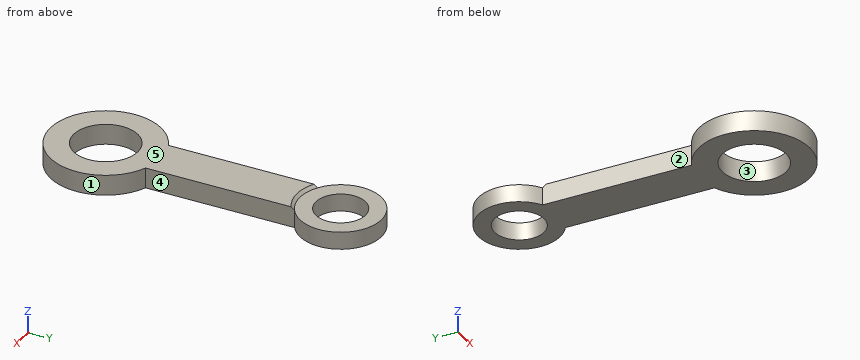
Autodesk Inventor part; units mm, degrees
ref_plane "YZ Plane" through (0, 0, 0) normal (1, 0, 0) x (0, 1, 0)
ref_plane "XZ Plane" through (0, 0, 0) normal (0, 1, 0) x (-1, 0, 0)
ref_plane "XY Plane" through (0, 0, 0) normal (0, 0, 1) x (1, 0, 0)
sketch "Sketch1" plane through (0, 0, 0) normal (0, 0, 1) x (1, 0, 0)
  line L0 (0, 0) -> (0, 80) construction
  circle A0 centre (0, 0) radius 11
  circle A1 centre (0, 80) radius 8.5
  line L1 (7.5, 17.4571) -> (-7.5, 17.4571)
  line L2 (-7.5, 17.4571) -> (-7.5, 68.1784)
  line L3 (-7.5, 68.1784) -> (7.5, 68.1784)
  line L4 (7.5, 68.1784) -> (7.5, 17.4571)
  line L5 (7.5, 17.4571) -> (-7.5, 68.1784) construction
  line L6 (-7.5, 17.4571) -> (7.5, 68.1784) construction
  arc A2 (7.5, 68.1784) -> (-7.5, 68.1784) centre (0, 80) ccw
  arc A3 (-7.5, 17.4571) -> (7.5, 17.4571) centre (0, 0) ccw
  point P0 (0, 42.8177)
  point P1 (0, 42.8177)
  dimension "d0" = 22
  dimension "d1" = 17
  dimension "d2" = 80
  dimension "d3" = 5.5
  dimension "d4" = 8
  dimension "d5" = 15
extrude "Extrusion1" add sketch "Sketch1" along normal blind 7
sketch "Sketch2" plane through (0, 0, 7) normal (0, 0, 1) x (1, 0, 0)
  circle A0 centre (0, 80) radius 8.5
  arc A1 (7.5, 68.1784) -> (-7.5, 68.1784) centre (0, 80) ccw
  circle A2 centre (0, 80) radius 14
extrude "Extrusion2" cut sketch "Sketch2" against normal blind 1
chamfer "Chamfer1" distance 1 angle 45 1 edges at (0, 66, 7)
properties part number "con rod"
Build history of the part. All positions in model axes, mm. Face numbers are marked on the shaded views. A direction names the side the tool comes from. Give positions to 0.01 mm unless a question says otherwise; leave off trailing zeros. Order: outer loops, then holes, each group sorted by start corner. A loop starts at its lowest first (then second) coordinate and runs counter-clockwise, first axis right, second up. Notation, with made-up numbers: M -20,75.5 L 2,75.5 A18 cw 2,99.5 Z; hole C 21,15.5 d8. An arc over 180 degrees is marked long. Put each result on its own line as item: value.
Item 1: Slice it at B-B, the plane y = 80. Write the cut outline in (x, z).
From the geometry:
outline: M -14,0 L -8.5,0 L -8.5,6 L -14,6 Z; M 8.5,0 L 14,0 L 14,6 L 8.5,6 Z
Item 2: Slice it at A-A, the plane x = 0. Give the number of separate pieces and of enclosed holes in the cut face, plus the area to 4 significant figures.
From the geometry:
separate pieces: 3
enclosed holes: 0
area: 506.5 mm2
Item 3: Slice it at C-C, the plane z = 3.5. Write the cut outline in (x, y).
From the geometry:
outline: M -7.5,17.46 A19 ccw long 7.5,17.46 L 7.5,68.18 A14 ccw long -7.5,68.18 Z; hole C 0,0 d22; hole C 0,80 d17
Item 4: 3-axis set-ups, long thin cutter, end or side, ignore diameter. For the marked faces 1 and 2: which of +Z, -Z, +X, -X, +Y, -Y reach the whole face in a straight line?
From the geometry:
face 1: +Z, -Z
face 2: +Z, -Z, -X
Item 5: Probe line 1 (Y direction, x = 0, z = 1.85); line 2 (Y direction, x = 7, z = 5); line 3 (X direction, y = 32, z = 1.75). List the from-to ranges inside material, lowest first. Write a range as [from, to].
From the geometry:
line 1: y = [-19, -11], [11, 71.5], [88.5, 94]
line 2: y = [-17.66, -8.49], [8.49, 75.18], [84.82, 92.12]
line 3: x = [-7.5, 7.5]
Item 6: Flat gauge pins, fed straight in: pin 1 Ø1.5 at (x, z) = (-1, 4.5) entering from +Y; pin 2 Ø10 at (x, y) = (-8, 35) entering from -Z; pin 3 Ø2 at (y, z) = (34.5, 5) entering from +X; pin 4 Ø3 at (x, z) = (13.5, 2) entering from -Y. Where does each tip first touch, or does it go through?
From the geometry:
pin 1: stops at y = 94
pin 2: stops at z = 0
pin 3: stops at x = 7.5
pin 4: stops at y = -14.73
Item 7: Slice it at D-D, the plane x = -12.5. Write the cut outline in (y, z), plus the area to 3 significant figures.
From the geometry:
outline: M -14.31,0 L 14.31,0 L 14.31,7 L -14.31,7 Z; M 73.7,0 L 86.3,0 L 86.3,6 L 73.7,6 Z
area: 276 mm2
Item 8: Two-plate mould, pull along Y, no slides. Class the marked faces 3, 4 and 5: +Y half, -Y half, draft (parallel to the pull), parting line (faces both ways), or undercut.
From the geometry:
face 3: undercut
face 4: undercut
face 5: draft
